Job drawing, mm, ordinate dimensions from the low corner. One solid piece. Coordinates: 2 decimals unless noted, no trailing zeros. Loops run counter-clockwise (first coordinate to the right, second up) from the corner with the lowest first, then second, coordinate; pieces in that order, holes last. Notation, with made-up numbers: (58, 29) -> (95, 29) arc R26 ccw to (95, 45) -> close; hole circle Ø7 at (8.5, 34). An arc over 180 degrees is marked (long way). Use one line per item in the form item = value. Start each with the question number.
(1) Band-saw the part on B-B on x = 18. Give the cut face in (y, z), then the cut area to 3 significant figures.
(2) Band-saw the part on A-A on y = 23. Give the cut face in (x, z), then the cut area to 3 significant figures.
(3) Band-saw the part on C-C on z = 4. Give the cut face in (x, y).
(4) Drill centre lines: L1, parallel to Y at x = 31, z = 4; L2, parallel to Y at x = 30, z = 2.75; L3, parallel to Z at x = 10, y = 14. Where is each one in solid material? Low to high. Write a range as [from, to].
(5) Pin check, flat tip, straight feed: P1, Ø3, axis at y = 23, z = 4, coming from the -X side. Stop position of the tip, or through.
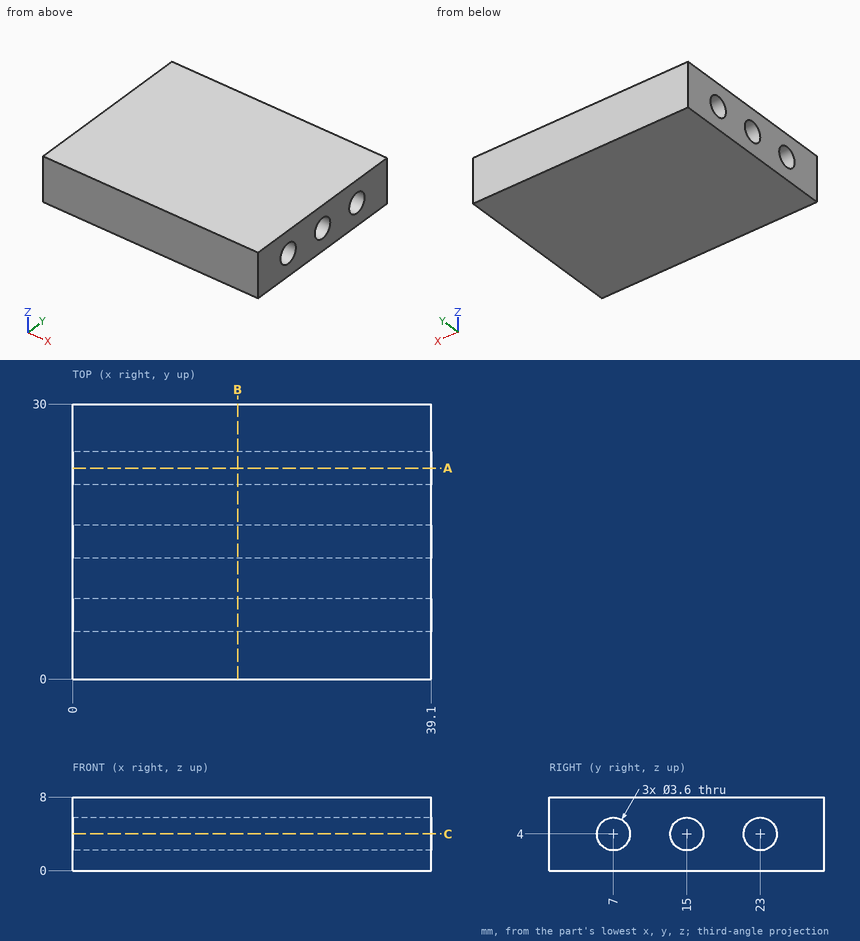
A:
q1.outline = (0, 0) -> (30, 0) -> (30, 8) -> (0, 8) -> close; hole circle Ø3.6 at (7, 4); hole circle Ø3.6 at (15, 4); hole circle Ø3.6 at (23, 4)
q1.area = 209 mm²
q2.outline = (0, 0) -> (39.1, 0) -> (39.1, 2.2) -> (0, 2.2) -> close; (0, 5.8) -> (39.1, 5.8) -> (39.1, 8) -> (0, 8) -> close
q2.area = 172 mm²
q3.outline = (0, 0) -> (39.1, 0) -> (39.1, 5.2) -> (0, 5.2) -> close; (0, 8.8) -> (39.1, 8.8) -> (39.1, 13.2) -> (0, 13.2) -> close; (0, 16.8) -> (39.1, 16.8) -> (39.1, 21.2) -> (0, 21.2) -> close; (0, 24.8) -> (39.1, 24.8) -> (39.1, 30) -> (0, 30) -> close
q4.L1 = [0, 5.2], [8.8, 13.2], [16.8, 21.2], [24.8, 30]
q4.L2 = [0, 5.7], [8.3, 13.7], [16.3, 21.7], [24.3, 30]
q4.L3 = [0, 2.5], [5.5, 8]
q5.P1 = through
